from build123d import *

# Parameters (mm, degrees)
CYLINDER081_R               = 1.9
CYLINDER081_DEPTH           = 20
BOX082_W                    = 3
BOX082_H                    = 24
BOX082_DEPTH                = 20
BOX082_PITCH_ANGLE          = -15
CYLINDER082_R               = 1.1
CYLINDER082_DEPTH           = 20
CYLINDER082_PLACEMENT_ANGLE = 75
CYLINDER083_R               = 1.1
CYLINDER083_DEPTH           = 20
CYLINDER083_PLACEMENT_ANGLE = 75
BOX080_W                    = 5
BOX080_H                    = 20
BOX080_DEPTH                = 15
BOX080_PITCH_ANGLE          = -15
BOX081_W                    = 16
BOX081_H                    = 20
BOX081_DEPTH                = 4
FILLET019_R                 = 5
FILLET021_R                 = 3
FILLET022_R                 = 3
FILLET023_R                 = 1.5


with BuildPart() as cylinder081:
    # Cylinder081 → Cylinder081 (new body)
    with BuildSketch(Plane(origin=(529, 40, -10), x_dir=(1, 0, 0), z_dir=(0, 0, 1))):
        Circle(CYLINDER081_R)
    extrude(amount=CYLINDER081_DEPTH)


with BuildPart() as cube054:
    # Box082 → Box082 (new body)
    with BuildSketch(Plane.XY):
        with Locations((1.5, 12)):
            Rectangle(BOX082_W, BOX082_H)
    extrude(amount=BOX082_DEPTH)


with BuildPart() as cube054_1:
    # Box082 pitch: moved
    add(cube054.part.rotate(Axis((0, 0, 0), (0, 1, 0)), BOX082_PITCH_ANGLE))


with BuildPart() as cube054_2:
    # Box082 placement: moved
    add(cube054_1.part.moved(Location((540, 28, 2))))


with BuildPart() as cylinder082:
    # Cylinder082 → Cylinder082 (new body)
    with BuildSketch(Plane.XY):
        Circle(CYLINDER082_R)
    extrude(amount=CYLINDER082_DEPTH)


with BuildPart() as cylinder082_1:
    # Cylinder082 placement: moved
    add(cylinder082.part.moved(Location((532, 35, 7.5))).rotate(Axis((532, 35, 7.5), (0, 1, 0)), CYLINDER082_PLACEMENT_ANGLE))


with BuildPart() as fusion090:
    # Cylinder083 → Cylinder083 (new body)
    with BuildSketch(Plane.XY):
        Circle(CYLINDER083_R)
    extrude(amount=CYLINDER083_DEPTH)


with BuildPart() as fusion090_1:
    # Cylinder083 placement: moved
    add(fusion090.part.moved(Location((532, 45, 7.5))).rotate(Axis((532, 45, 7.5), (0, 1, 0)), CYLINDER083_PLACEMENT_ANGLE))

    # Fusion090: union Cylinder082
    add(cylinder082_1.part)


with BuildPart() as fusion090_2:
    # Fusion090 placement: moved
    add(fusion090_1.part.moved(Location((0, 0, 4))))


with BuildPart() as cube052:
    # Box080 → Box080 (new body)
    with BuildSketch(Plane.XY):
        with Locations((2.5, 10)):
            Rectangle(BOX080_W, BOX080_H)
    extrude(amount=BOX080_DEPTH)


with BuildPart() as cube052_1:
    # Box080 pitch: moved
    add(cube052.part.rotate(Axis((0, 0, 0), (0, 1, 0)), BOX080_PITCH_ANGLE))


with BuildPart() as cube052_2:
    # Box080 placement: moved
    add(cube052_1.part.moved(Location((536, 30, 2))))


with BuildPart() as rear_door_closure_lock:
    # Box081 → Box081 (new body)
    with BuildSketch(Plane(origin=(524, 30, 2), x_dir=(1, 0, 0), z_dir=(0, 0, 1))):
        with Locations((8, 10)):
            Rectangle(BOX081_W, BOX081_H)
    extrude(amount=BOX081_DEPTH)

    # Fusion095: union Cube052
    add(cube052_2.part)

    # Cut102: cut Fusion090
    add(fusion090_2.part, mode=Mode.SUBTRACT)

    # Cut103: cut Cube054
    add(cube054_2.part, mode=Mode.SUBTRACT)

    # Cut104: cut Cylinder081
    add(cylinder081.part, mode=Mode.SUBTRACT)

    # Fillet019
    fillet019_edges = [rear_door_closure_lock.edges().sort_by_distance(p)[0] for p in [
        (524, 30, 4),
        (524, 50, 4),
    ]]
    fillet(fillet019_edges, radius=FILLET019_R)

    # Fillet021
    fillet021_edges = [rear_door_closure_lock.edges().sort_by_distance(p)[0] for p in [
        (534.928203, 40, 6),
    ]]
    fillet(fillet021_edges, radius=FILLET021_R)

    # Fillet022
    fillet022_edges = [rear_door_closure_lock.edges().sort_by_distance(p)[0] for p in [
        (532.117714, 40, 16.488887),
    ]]
    fillet(fillet022_edges, radius=FILLET022_R)

    # Fillet023
    fillet023_edges = [rear_door_closure_lock.edges().sort_by_distance(p)[0] for p in [
        (524, 40, 6),
        (524, 40, 2),
    ]]
    fillet(fillet023_edges, radius=FILLET023_R)


solid = rear_door_closure_lock.part
Can you work these out from the model? Positions are in its coordinate system, mm. A direction names the side the tool comes from. Coordinates: 2 decimals unless noted, no trailing zeros. Write each loop counter-clockwise with the first axis right and the second up, starting at its lowest first coordinate (ties: lowest second). Pieces come first, ordered by that corner, then holes. Notation, with made-up numbers: (61, -30) - (80, -30) arc R23 ccw to (80, -22) - close; hole circle Ø9 at (-15.75, -38.5). An arc over 180 degrees is marked (long way). Return JSON: item names as keys, results as strings. Group by question number.
Item 1: Which directions (+Z, -Z, +X, -X, +Y, -Y) give clear straight access to the entire face, cutting with the end or side of a thin tool? Please do faces 4 (the face through (533.81, 49.55, 11.82)), 5 (the face through (533.826, 30.451, 11.768)), 6 (the face through (530, 30.45, 5.57)), 7 (the face through (533.18, 40.12, 15.84)).
Item 2: I'm going to push flat-ended pins straight in: pin 1 Ø6 at (x, y) = (527.5, 37.5) entering from +Z; pin 2 Ø6 at (y, z) = (40.5, 5.5) entering from +X; pin 3 Ø1.5 at (y, z) = (37, 5.5) entering from -X. Where does each tip first touch, or does it pass through?
Item 3: We'd pull the mould along X, two halves only. Please class faces 1 (the face through (535.5, 49.5, 17)), 2 (the face through (530.02, 49.55, 5.57)), 3 (the face through (530.755, 39.272, 3.972)): pulls with the +X half, pulls with the -X half, needs draft (parallel to the pull), parting line crosses it, or undercut.
Item 4: If we section it at B-B (y = 35.5): Write out the boundary of the cut face in (x, z), then the cut area to 3 significant figures.
Item 5: If we section it at A-A (y = 40): Write out the boundary of the cut face in (x, z).
Item 6: Please list where these lines run through material, in increasing order: probe 1 along Y at (x, z) = (529, 3.7); probe 2 along Y at (x, z) = (534.5, 12); probe 3 along X at (y, z) = (40, 5).
Return value:
{
 "1": {"face 4": "-X, +Y", "face 5": "-X, -Y", "face 6": "+Z, -X, -Y", "face 7": "-X, +Y, -Y"},
 "2": {"pin 1": "stops at z = 6", "pin 2": "stops at x = 539.87", "pin 3": "stops at x = 524.02"},
 "3": {"face 1": "pulls with the -X half", "face 2": "needs draft", "face 3": "undercut"},
 "4": {"outline": "(524, 3.5) arc R1.5 ccw to (525.5, 2) - (540, 2) - (537.34, 11.92) - (533.61, 10.92) - (533.92, 9.78) arc R3 cw to (531.02, 6) - (525.5, 6) arc R1.5 ccw to (524, 4.5) - close; (532.89, 13.59) - (533.1, 12.81) - (536.84, 13.81) - (535.85, 17.49) - (535.02, 17.27) arc R3 ccw to start", "area": "98.8 mm^2"},
 "5": {"outline": "(524, 3.5) arc R1.5 ccw to (525.5, 2) - (527.1, 2) - (527.1, 6) - (525.5, 6) arc R1.5 ccw to (524, 4.5) - close; (530.9, 2) - (540, 2) - (535.85, 17.49) - (535.02, 17.27) arc R3 ccw to (532.89, 13.59) - (533.92, 9.78) arc R3 cw to (531.02, 6) - (530.9, 6) - close"},
 "6": {"probe 1": "y = 30 to 38.1, 41.9 to 50", "probe 2": "y = 30.04 to 33.91, 36.09 to 43.91, 46.09 to 49.96", "probe 3": "x = 524.09 to 527.1, 530.9 to 539.2"}
}
